Here's how the part is built. I have some questions about the finished solid (model axes, mm). A direction names the side the tool comes from. Round coordinates to 2 decimals unless told otherwise and drop trailing zeros. Loops run counter-clockwise (first coordinate to the right, second up) from the corner with the lowest first, then second, coordinate; pieces in that order, holes last. Notation, with made-up numbers: M 24,36 L 43,36 A27 ccw 43,58 Z; hole C 81,-2.75 d10. An arc over 180 degrees is marked long. Answer as a JSON object with one key per item and string values.
from build123d import *

# Parameters (mm, degrees)
SKETCH1_W             = 6
SKETCH1_H             = 12
EXTRUDE1_DEPTH        = 8
SKETCH3_W             = 4
SKETCH3_H             = 8.6
EXTRUDE2_DEPTH        = 1
SKETCH2_R             = 1.25
EXTRUDE3_DEPTH        = 6
EXTRUDE4_DEPTH        = 4
SKETCH8_R             = 5.25
EXTRUDE7_DEPTH        = 1
SKETCH7_R             = 1
EXTRUDE6_DEPTH        = 4
CIRPATTERN1_COUNT     = 3
SKETCH9_R             = 2
EXTRUDE8_DEPTH        = 3
M3_TAPPED_HOLE1_D     = 2.5
M3_TAPPED_HOLE1_DEPTH = 6
M3_TAPPED_HOLE1_TIP   = 0.751075774
FILLET1_R             = 4


with BuildPart() as part:
    # Sketch1 → Extrude1 (new body)
    with BuildSketch(Plane.XY):
        with Locations((1, 0)):
            Rectangle(SKETCH1_W, SKETCH1_H)
    extrude(amount=EXTRUDE1_DEPTH)

    # Sketch3 → Extrude2 (add)
    with BuildSketch(Plane.XY.offset(8)):
        Rectangle(SKETCH3_W, SKETCH3_H)
    extrude(amount=EXTRUDE2_DEPTH)

    # Sketch2 → Extrude3 (cut)
    with BuildSketch(Plane(origin=(0, 0, 0), x_dir=(-1, 0, 0), z_dir=(0, 0, -1))):
        with Locations((-1, 3)):
            Circle(SKETCH2_R)
        with Locations((-1, -3)):
            Circle(SKETCH2_R)
    extrude(amount=-EXTRUDE3_DEPTH, mode=Mode.SUBTRACT)

    # Sketch4 → Extrude4 (add)
    with BuildSketch(Plane(origin=(2, 0, 0), x_dir=(0, 0, -1), z_dir=(1, 0, 0))):
        with BuildLine():
            Line((-9.900455543, 6), (-8, 6))
            Line((-8, 6), (-8, -6))
            Line((-8, -6), (-9.900455543, -6))
            ThreePointArc((-9.900455543, -6), (-30.12, 0), (-9.900455543, 6))
        make_face()
    extrude(amount=-EXTRUDE4_DEPTH)

    # Sketch8 → Extrude7 (cut)
    with BuildSketch(Plane(origin=(2, 0, 0), x_dir=(0, 0, -1), z_dir=(1, 0, 0))):
        with Locations(Location((-19.12, 0, 0), (0, 0, 90))):
            Circle(SKETCH8_R)
    extrude(amount=-EXTRUDE7_DEPTH, mode=Mode.SUBTRACT)

    # Sketch7 → Extrude6 (cut)
    with BuildSketch(Plane.ZY.offset(2)):
        with Locations(Location((19.12, -7.5, 0), (0, 0, 270))):
            Circle(SKETCH7_R)
    extrude6 = extrude(amount=-EXTRUDE6_DEPTH, mode=Mode.SUBTRACT)

    # CirPattern1: Extrude6 ×3 about axis
    cirpattern1_axis = Axis((0, 0, 18.12), (1, 0, 0))
    for i in range(1, CIRPATTERN1_COUNT):
        add(extrude6.rotate(cirpattern1_axis, i * 360 / CIRPATTERN1_COUNT), mode=Mode.SUBTRACT)

    # Sketch9 → Extrude8 (cut)
    with BuildSketch(Plane(origin=(1, 0, 0), x_dir=(0, 0, -1), z_dir=(1, 0, 0))):
        with Locations(Location((-19.12, 0, 0), (0, 0, 90))):
            Circle(SKETCH9_R)
    extrude(amount=-EXTRUDE8_DEPTH, mode=Mode.SUBTRACT)

    # M3 Tapped Hole1
    with Locations(Plane(origin=(1, 3, 0), x_dir=(-1, 0, 0), z_dir=(0, 0, -1))):
        with Locations((0, 0), (0, -6)):
            Hole(M3_TAPPED_HOLE1_D / 2, depth=M3_TAPPED_HOLE1_DEPTH)
            with Locations((0, 0, -(M3_TAPPED_HOLE1_DEPTH + M3_TAPPED_HOLE1_TIP / 2))):  # 118° drill point
                Cone(0, M3_TAPPED_HOLE1_D / 2, M3_TAPPED_HOLE1_TIP, mode=Mode.SUBTRACT)

    # Fillet1
    # the kernel refuses this fillet: 4 mm, written as the material it adds along each edge
    with BuildSketch(Plane(origin=(6.901988576, -6, 9.900455543), x_dir=(0, 0, -1), z_dir=(-1, 0, 0))) as fillet1_piece_1_section:
        with BuildLine():
            CenterArc((1.96079543, 4), FILLET1_R, 221.810314896, 48.189685104)
            ThreePointArc((-1.02062854, 1.333333333), (-0.484835824, 0.686169688), (0, 0))
            Line((0, 0), (1.96079543, 0))
        make_face()
    fillet1_piece_1 = extrude(amount=8.901988576, mode=Mode.PRIVATE)
    fillet1_piece_1 = split(fillet1_piece_1, bisect_by=Plane(origin=(4, -5.96007597, 7.969858609), z_dir=(-1, 0, 0)), keep=Keep.TOP, mode=Mode.PRIVATE)
    fillet1_piece_1 = split(fillet1_piece_1, bisect_by=Plane(origin=(3, -5.96007597, 8), z_dir=(0, 0, -1)), keep=Keep.TOP, mode=Mode.PRIVATE)
    fillet1_piece_1 = split(fillet1_piece_1, bisect_by=Plane(origin=(2, -5.96007597, 7.969858609), z_dir=(1, 0, 0)), keep=Keep.TOP, mode=Mode.PRIVATE)
    add(fillet1_piece_1)
    with BuildSketch(Plane(origin=(2, -6, 9.900455543), x_dir=(0, 0, -1), z_dir=(-1, 0, 0))) as fillet1_piece_2_section:
        with BuildLine():
            CenterArc((1.96079543, 4), FILLET1_R, 221.810314896, 48.189685104)
            ThreePointArc((-1.02062854, 1.333333333), (-0.484835824, 0.686169688), (0, 0))
            Line((0, 0), (1.96079543, 0))
        make_face()
    fillet1_piece_2 = extrude(amount=4, mode=Mode.PRIVATE)
    fillet1_piece_2 = split(fillet1_piece_2, bisect_by=Plane(origin=(0, -5.96007597, 8), z_dir=(0, 0, -1)), keep=Keep.TOP, mode=Mode.PRIVATE)
    add(fillet1_piece_2)
    with BuildSketch(Plane(origin=(2, -6, 9.900455543), x_dir=(0, 0, -1), z_dir=(-1, 0, 0))) as fillet1_piece_3_section:
        with BuildLine():
            CenterArc((1.96079543, 4), FILLET1_R, 221.810314896, 48.189685104)
            ThreePointArc((-1.02062854, 1.333333333), (-0.484835824, 0.686169688), (0, 0))
            Line((0, 0), (1.96079543, 0))
        make_face()
    fillet1_piece_3 = extrude(amount=4, mode=Mode.PRIVATE)
    fillet1_piece_3 = split(fillet1_piece_3, bisect_by=Plane(origin=(0, -6.284176822, 8), z_dir=(0, 0, 1)), keep=Keep.TOP, mode=Mode.PRIVATE)
    add(fillet1_piece_3)
    with BuildSketch(Plane(origin=(6.901988576, 6, 9.900455543), x_dir=(0, 0, -1), z_dir=(-1, 0, 0))) as fillet1_piece_4_section:
        with BuildLine():
            CenterArc((1.96079543, -4), FILLET1_R, 90, 48.189685104)
            ThreePointArc((-1.02062854, -1.333333333), (-0.484835824, -0.686169688), (0, 0))
            Line((0, 0), (1.96079543, 0))
        make_face()
    fillet1_piece_4 = extrude(amount=8.901988576, mode=Mode.PRIVATE)
    fillet1_piece_4 = split(fillet1_piece_4, bisect_by=Plane(origin=(2, 5.96007597, 7.969858609), z_dir=(1, 0, 0)), keep=Keep.TOP, mode=Mode.PRIVATE)
    fillet1_piece_4 = split(fillet1_piece_4, bisect_by=Plane(origin=(3, 5.96007597, 8), z_dir=(0, 0, -1)), keep=Keep.TOP, mode=Mode.PRIVATE)
    fillet1_piece_4 = split(fillet1_piece_4, bisect_by=Plane(origin=(4, 5.96007597, 7.969858609), z_dir=(-1, 0, 0)), keep=Keep.TOP, mode=Mode.PRIVATE)
    add(fillet1_piece_4)
    with BuildSketch(Plane(origin=(2, 6, 9.900455543), x_dir=(0, 0, -1), z_dir=(-1, 0, 0))) as fillet1_piece_5_section:
        with BuildLine():
            CenterArc((1.96079543, -4), FILLET1_R, 90, 48.189685104)
            ThreePointArc((-1.02062854, -1.333333333), (-0.484835824, -0.686169688), (0, 0))
            Line((0, 0), (1.96079543, 0))
        make_face()
    fillet1_piece_5 = extrude(amount=4, mode=Mode.PRIVATE)
    fillet1_piece_5 = split(fillet1_piece_5, bisect_by=Plane(origin=(0, 5.96007597, 8), z_dir=(0, 0, -1)), keep=Keep.TOP, mode=Mode.PRIVATE)
    add(fillet1_piece_5)
    with BuildSketch(Plane(origin=(2, 6, 9.900455543), x_dir=(0, 0, -1), z_dir=(-1, 0, 0))) as fillet1_piece_6_section:
        with BuildLine():
            CenterArc((1.96079543, -4), FILLET1_R, 90, 48.189685104)
            ThreePointArc((-1.02062854, -1.333333333), (-0.484835824, -0.686169688), (0, 0))
            Line((0, 0), (1.96079543, 0))
        make_face()
    fillet1_piece_6 = extrude(amount=4, mode=Mode.PRIVATE)
    fillet1_piece_6 = split(fillet1_piece_6, bisect_by=Plane(origin=(0, 6.284176822, 8), z_dir=(0, 0, 1)), keep=Keep.TOP, mode=Mode.PRIVATE)
    add(fillet1_piece_6)


solid = part.part
Item 1: I want a section at C-C on z = 4.5. List the corners of the cut face in (x, y) for me, plus the area to 3 significant figures.
Solution:
{"outline": "M -2,-6 L 4,-6 L 4,6 L -2,6 Z; hole C 1,-3 d2.5; hole C 1,3 d2.5", "area": "62.2 mm2"}
Item 2: We'd pull the mould along Y, two halves only. Please class faces 1 (the face through (1, 6, 4)), 2 (the face through (-0.03, 4.08, 24.96)), 3 (the face through (1, 0, 0)): +Y half, -Y half, draft (parallel to the pull), parting line (faces both ways), or undercut.
Solution:
{"face 1": "+Y half", "face 2": "undercut", "face 3": "draft"}
Item 3: If I drill on L1, parallel to Y at x = 1, z = 1.4; L2, parallel to Y at x = 0.55, z = 19; L3, parallel to Z at x = 1.75, y = 2.75, over which ranges is the centre line in solid material (lowest first)? Write a range as from..to.
Solution:
{"L1": "y = -6..-4.25, -1.75..1.75, 4.25..6", "L2": "y = -11..-8.49, -6.51..-2, 2..11", "L3": "z = 6.28..10.13, 12.12..14.65, 23.59..29.77"}
Item 4: I want a section at B-B on y = 0. List the corners of the cut face in (x, z) for me, plus the area to 3 significant figures.
Solution:
{"outline": "M -2,0 L 4,0 L 4,8 L 2,8 L 2,13.87 L 1,13.87 L 1,17.12 L -2,17.12 Z; M -2,21.12 L 1,21.12 L 1,24.37 L 2,24.37 L 2,30.12 L -2,30.12 Z", "area": "114 mm2"}
Item 5: I want a section at D-D on x = -1.6. List the corners of the cut face in (y, z) for me.
Solution:
{"outline": "M -7.33,10.92 A4 cw -6,7.94 L -6,0 L 6,0 L 6,7.94 A4 cw 7.33,10.92 A11 ccw long Z; hole C -7.5,19.12 d2; hole C 0,19.12 d4; hole C 2.88,11.12 d2; hole C 4.62,24.12 d2"}
Item 6: For P1, Ø2.5, axis at y = 4.62, z = 24.12, coming from the +X side; P2, Ø2, axis at x = 1, y = -3, coming from the +Z side; P3, Ø12, axis at y = 0, z = 19.12, coming from the -X side; P4, Ø3, axis at x = 2.5, y = -2.5, coming from the +Z side, each with a flat end and sliding along its axis, tell me the tip position at first contact or that it passes through.
Solution:
{"P1": "stops at x = 2", "P2": "stops at z = 29.94", "P3": "stops at x = -2", "P4": "stops at z = 30.07"}
Item 7: I want a section at A-A on z = 19.12. List the corners of the cut face in (x, y) for me, plus the area to 3 significant figures.
Solution:
{"outline": "M -2,-11 L 2,-11 L 2,-8.5 L -2,-8.5 Z; M -2,-6.5 L 2,-6.5 L 2,-5.25 L 1,-5.25 L 1,-2 L -2,-2 Z; M -2,2 L 1,2 L 1,5.25 L 2,5.25 L 2,11 L -2,11 Z", "area": "57.5 mm2"}
Item 8: For faces 4 (the face through (1, -6, 4)), 5 (the face through (1.921, -2.155, 2.958)), 6 (the face through (3, 0, 8)), 7 (the face through (1, 2.3, 19.2)), which set-ups out of +Z, -Z, +X, -X, +Y, -Y let a thin tool reach every point of the face, with its end or its side?
Solution:
{"face 4": "-Z, +X, -X, -Y", "face 5": "-Z", "face 6": "+Z, +X, +Y, -Y", "face 7": "+X"}
